from build123d import *

# Parameters (mm, degrees)
F0_W     = 5
F0_H     = 20.3830654012
F0_W_2   = 3
F1_DEPTH = 50
F2_R     = 2.7
F3_DEPTH = 25
F4_R     = 12.7
F4_R_2   = 2.7
F5_DEPTH = 12
F6_SIZE  = 5.99999
F4_R_3   = 2.8
F7_DEPTH = 25
F8_R     = 2


# Not quite as in the source:
# - a fillet or chamfer is up to 0.001 mm smaller than in the source, because OpenCascade refuses the exact size


with BuildPart() as f1:
    # F0 (on Top) → F1 (new body)
    with BuildSketch(Plane.XY):
        with BuildLine():
            ThreePointArc((-34.9838541491, 0.5), (-26.9998696897, 7.7459624856), (-19.5, 0))
            ThreePointArc((-19.5, 0), (-26.9998696897, -7.7459624856), (-34.9838541491, -0.5))
            Line((-34.9838541491, -0.5), (-47.5, -0.5))
            Line((-47.5, -0.5), (-47.5, -10.0949762179))
            Line((-47.5, -10.0949762179), (47.5, -10.0949762179))
            Line((47.5, -10.0949762179), (47.5, -0.5))
            Line((47.5, -0.5), (34.9838541491, -0.5))
            ThreePointArc((34.9838541491, -0.5), (19.5, 0), (34.9838541491, 0.5))
            Line((34.9838541491, 0.5), (47.5, 0.5))
            Line((47.5, 0.5), (47.5, 10.0949762179))
            Line((47.5, 10.0949762179), (9.5, 10.0949762179))
            Line((9.5, 10.0949762179), (4.5, 10.0949762179))
            Line((4.5, 10.0949762179), (3, 10.0949762179))
            Line((3, 10.0949762179), (0, 10.0949762179))
            Line((0, 10.0949762179), (-3, 10.0949762179))
            Line((-3, 10.0949762179), (-4.5, 10.0949762179))
            Line((-4.5, 10.0949762179), (-9.5, 10.0949762179))
            Line((-9.5, 10.0949762179), (-47.5, 10.0949762179))
            Line((-47.5, 10.0949762179), (-47.5, 0.5))
            Line((-47.5, 0.5), (-34.9838541491, 0.5))
        make_face()
        with Locations((-7, 20.2865089185)):
            Rectangle(F0_W, F0_H)
        with Locations((-1.5, 20.2865089185)):
            Rectangle(F0_W_2, F0_H)
        with Locations((1.5, 20.2865089185)):
            Rectangle(F0_W_2, F0_H)
    extrude(amount=F1_DEPTH)

    # F2 (on face) → F3 (cut)
    with BuildSketch(Plane.YZ.offset(3)):
        with Locations((20.2865089185, 37.5)):
            Circle(F2_R)
        with Locations((20.2865089185, 12.5)):
            Circle(F2_R)
    extrude(amount=-F3_DEPTH, mode=Mode.SUBTRACT)

    # F4 (on face) → F5 (join)
    with BuildSketch(Plane.XZ.offset(10.0949762179)):
        with Locations((-22, 25)):
            Circle(F4_R)
        with Locations((-22, 25)):
            Circle(F4_R_2, mode=Mode.SUBTRACT)
        with Locations((22, 25)):
            Circle(F4_R)
        with Locations((22, 25)):
            Circle(F4_R_2, mode=Mode.SUBTRACT)
    extrude(amount=F5_DEPTH)

    # F6 (size 6 in the source; OpenCascade refuses exactly that, so slightly less here)
    f6_edges = [f1.edges().sort_by_distance(p)[0] for p in [
        (-34.7, -10.094976, 25),
        (-34.7, -22.094976, 25),
        (9.3, -22.094976, 25),
        (9.3, -10.094976, 25),
    ]]
    chamfer(f6_edges, length=F6_SIZE)

    # F4 (on face) → F7 (cut)
    with BuildSketch(Plane.XZ.offset(10.0949762179)):
        with Locations((-40.5, 37.5)):
            Circle(F4_R_3)
        with Locations((-40.5, 12.5)):
            Circle(F4_R_3)
        with Locations((40.5, 37.5)):
            Circle(F4_R_3)
        with Locations((40.5, 12.5)):
            Circle(F4_R_3)
    extrude(amount=-F7_DEPTH, mode=Mode.SUBTRACT)

    # F8
    f8_edges = [f1.edges().sort_by_distance(p)[0] for p in [
        (-28.70001, -22.094976, 25),
        (-24.7, -22.094976, 25),
        (15.29999, -22.094976, 25),
        (19.3, -22.094976, 25),
    ]]
    fillet(f8_edges, radius=F8_R)


solid = f1.part
The model under review builds one solid part; all positions refer to its coordinate system, in mm. A direction names the side the tool comes from. Coordinates: 2 decimals unless noted, no trailing zeros. Write each loop counter-clockwise with the first axis right and the second up, starting at its lowest first coordinate (ties: lowest second). Pieces come first, ordered by that corner, then holes. Notation, with made-up numbers: (69, 68.25) - (111, 68.25) arc R15 cw to (111, 76.25) - close; hole circle Ø8 at (-10, -6.75). An arc over 180 degrees is marked (long way). Answer as a JSON object with one key per item and string values. Group by question number.
1. Add section A-A (y = 3.5). Give the boundary of the cut face in (x, z), plus the area to 3 significant figures.
2. Clearance check with flat-ended pins moving along their axes: pin 1 Ø6 at (y, z) = (16, 33.5) entering from -X; pin 2 Ø1.6 at (x, z) = (-22.5, 24.5) entering from -Y (3 decimals); pin 3 Ø1 at (x, z) = (37, 17.5) entering from +Y (3 decimals). State where each tip first meets the part, or that it passes through.
3. To check wall thickness, follow probe 1 along Z at (x, y) = (-40.5, -4.75); probe 2 along X at (y, z) = (13, 47.5); probe 3 along Y at (x, z) = (-37, 40.5). State the ranges of each line that lie inside material, in increasing order.
4. Add section C-C (y = 20). Give the boundary of the cut face in (x, z).
5. Add section D-D (x = 0). Give the boundary of the cut face in (y, z).
6. Mouldability with a two-part tool opening along Y and no side actions: class faces 1 (the face through (-41, 0.5, 25)), 2 (the face through (22, -10.095, 25)), 3 (the face through (39.893, -5.365, 34.767)) as pulls with the +Y half, pulls with the -Y half, needs draft (parallel to the pull), parting line crosses it, or undercut.
7. Machinability: for faces 4 (the face through (-9.5, 20, 25)), 5 (the face through (-3, 20, 25)), 6 (the face through (41, 0.5, 25)), 7 (the face through (-20.548, -15.025, 27.277)), which of the approach directions +Z, -Z, +X, -X, +Y, -Y give a long, thin tool a straight path to every point of the face, cutting with its end or side? Answer none if there is none.
Findings:
{
 "1": {"outline": "(-47.5, 0) - (-34.16, 0) - (-34.16, 50) - (-47.5, 50) - close; (-20.34, 0) - (20.34, 0) - (20.34, 50) - (-20.34, 50) - close; (34.16, 0) - (47.5, 0) - (47.5, 50) - (34.16, 50) - close; hole circle Ø5.6 at (-40.5, 12.5); hole circle Ø5.6 at (-40.5, 37.5); hole circle Ø5.6 at (40.5, 12.5); hole circle Ø5.6 at (40.5, 37.5)", "area": "3,270 mm²"},
 "2": {"pin 1": "x = -9.5", "pin 2": "y = -10.095", "pin 3": "y = 10.095"},
 "3": {"probe 1": "0 to 9.7, 15.3 to 34.7, 40.3 to 50", "probe 2": "-9.5 to -4.5, -3 to 3", "probe 3": "-10.09 to -0.5, 0.5 to 10.09"},
 "4": {"outline": "(-9.5, 0) - (-4.5, 0) - (-4.5, 9.82) - (-9.5, 9.82) - close; (-9.5, 15.18) - (-4.5, 15.18) - (-4.5, 34.82) - (-9.5, 34.82) - close; (-9.5, 40.18) - (-4.5, 40.18) - (-4.5, 50) - (-9.5, 50) - close; (-3, 0) - (3, 0) - (3, 9.82) - (-3, 9.82) - close; (-3, 15.18) - (3, 15.18) - (3, 34.82) - (-3, 34.82) - close; (-3, 40.18) - (3, 40.18) - (3, 50) - (-3, 50) - close"},
 "5": {"outline": "(-10.09, 0) - (30.48, 0) - (30.48, 50) - (-10.09, 50) - close; hole circle Ø5.4 at (20.29, 12.5); hole circle Ø5.4 at (20.29, 37.5)"},
 "6": {"face 1": "undercut", "face 2": "pulls with the -Y half", "face 3": "needs draft"},
 "7": {"face 4": "+Z, -Z, -X, +Y", "face 5": "+Z, -Z, +Y", "face 6": "+Z, -Z, +X", "face 7": "-Y"}
}
